from build123d import *

# Parameters (mm, degrees)
BOSS_EXTRUDE1_DEPTH   = 30
FILLET1_R             = 10
CHAMFER1_SIZE         = 2
SKETCH3_R             = 1.9
CUT_EXTRUDE1_DEPTH    = 32.825
CHAMFER2_SIZE         = 2
CHAMFER2_SIZE2        = 0.352653961
CHAMFER2_PART_2_SIZE  = 2
CHAMFER2_PART_2_SIZE2 = 0.352653961
CHAMFER2_PART_3_SIZE  = 2
CHAMFER2_PART_3_SIZE2 = 0.352653961
CHAMFER2_PART_4_SIZE  = 2
CHAMFER2_PART_4_SIZE2 = 0.352653961


with BuildPart() as part:
    # Sketch1 → Boss-Extrude1 (new body)
    with BuildSketch(Plane.XY):
        with BuildLine():
            Line((0, 3.175), (0, 0))
            ThreePointArc((0, 0), (10.672667654, 4.397249215), (15.150137433, 15.036511402))
            ThreePointArc((15.150137433, 15.036511402), (20.018255831, 19.849965642), (24.85, 15))
            Line((24.85, 15), (24.85, 7.575))
            ThreePointArc((24.85, 7.575), (32.425, 0), (40, 7.575))
            Line((40, 7.575), (40, 15))
            ThreePointArc((40, 15), (25.241541186, 34.300938992), (2.747375401, 25.116666667))
            ThreePointArc((2.747375401, 25.116666667), (-0.908189135, 21.497922919), (-5.878936899, 20.175))
            Line((-5.878936899, 20.175), (-40, 20.175))
            Line((-40, 20.175), (-40, 3.175))
            Line((-40, 3.175), (0, 3.175))
        make_face()
    extrude(amount=BOSS_EXTRUDE1_DEPTH)

    # Fillet1
    fillet1_edges = [part.edges().sort_by_distance(p)[0] for p in [
        (-40, 11.675, 0),
        (-40, 11.675, 30),
    ]]
    fillet(fillet1_edges, radius=FILLET1_R)

    # Chamfer1
    chamfer1_edges = [part.edges().sort_by_distance(p)[0] for p in [
        (-17.939468449, 20.175, 0),
        (-0.908189135, 21.497922919, 0),
        (25.241541186, 34.300938992, 0),
        (40, 11.2875, 0),
        (10.672667654, 4.397249215, 30),
        (32.425, 0, 0),
        (24.85, 11.2875, 0),
        (20.018255831, 19.849965642, 0),
        (10.672667654, 4.397249215, 0),
        (0, 1.5875, 0),
        (20.018255831, 19.849965642, 30),
        (24.85, 11.2875, 30),
        (32.425, 0, 30),
        (40, 11.2875, 30),
        (25.241541186, 34.300938992, 30),
        (-40, 3.175, 15),
        (-40, 20.175, 15),
        (-15, 3.175, 0),
        (-15, 3.175, 30),
        (-37.071067812, 3.175, 27.071067812),
        (-0.908189135, 21.497922919, 30),
        (-37.071067812, 3.175, 2.928932188),
        (-37.071067812, 20.175, 27.071067812),
        (-37.071067812, 20.175, 2.928932188),
        (-17.939468449, 20.175, 30),
        (0, 1.5875, 30),
    ]]
    chamfer(chamfer1_edges, length=CHAMFER1_SIZE)

    # Sketch3 → Cut-Extrude1 (cut, through all)
    with BuildSketch(Plane.XZ.offset(-3.175)):
        with Locations((-30, 20)):
            Circle(SKETCH3_R)
        with Locations((-15, 20)):
            Circle(SKETCH3_R)
        with Locations((-15, 10)):
            Circle(SKETCH3_R)
        with Locations((-30, 10)):
            Circle(SKETCH3_R)
    extrude(amount=-CUT_EXTRUDE1_DEPTH, mode=Mode.SUBTRACT)

    # Chamfer2
    chamfer2_edges = [part.edges().sort_by_distance(p)[0] for p in [
        (-31.9, 3.175, 10),
    ]]
    chamfer2_side = [part.faces().sort_by_distance(p)[0] for p in [
        (-31.9, 11.675, 10),
    ]]
    chamfer(chamfer2_edges, length=CHAMFER2_SIZE, length2=CHAMFER2_SIZE2, reference=chamfer2_side[0])

    # Chamfer2 part 2
    chamfer2_part_2_edges = [part.edges().sort_by_distance(p)[0] for p in [
        (-16.9, 3.175, 10),
    ]]
    chamfer2_part_2_side = [part.faces().sort_by_distance(p)[0] for p in [
        (-16.9, 11.675, 10),
    ]]
    chamfer(chamfer2_part_2_edges, length=CHAMFER2_PART_2_SIZE, length2=CHAMFER2_PART_2_SIZE2, reference=chamfer2_part_2_side[0])

    # Chamfer2 part 3
    chamfer2_part_3_edges = [part.edges().sort_by_distance(p)[0] for p in [
        (-16.9, 3.175, 20),
    ]]
    chamfer2_part_3_side = [part.faces().sort_by_distance(p)[0] for p in [
        (-16.9, 11.675, 20),
    ]]
    chamfer(chamfer2_part_3_edges, length=CHAMFER2_PART_3_SIZE, length2=CHAMFER2_PART_3_SIZE2, reference=chamfer2_part_3_side[0])

    # Chamfer2 part 4
    chamfer2_part_4_edges = [part.edges().sort_by_distance(p)[0] for p in [
        (-31.9, 3.175, 20),
    ]]
    chamfer2_part_4_side = [part.faces().sort_by_distance(p)[0] for p in [
        (-31.9, 11.675, 20),
    ]]
    chamfer(chamfer2_part_4_edges, length=CHAMFER2_PART_4_SIZE, length2=CHAMFER2_PART_4_SIZE2, reference=chamfer2_part_4_side[0])


solid = part.part
Read the model definition and answer for the solid it produces. Units are mm, in the model's axes. A direction names the side the tool comes from. Coordinates: 2 decimals unless noted, no trailing zeros. Write each loop counter-clockwise with the first axis right and the second up, starting at its lowest first coordinate (ties: lowest second). Pieces come first, ordered by that corner, then holes. Notation, with made-up numbers: (23.25, 24.25) -> (70.25, 24.25) arc R14 ccw to (70.25, 46.25) -> close; hole circle Ø10 at (71.25, -24). An arc over 180 degrees is marked (long way). Return JSON: item names as keys, results as strings.
(1) Consider line 1 along Z through (x, y) = (-15, 10.25); line 2 along Y through (x, z) = (-35, 7.5) (3 decimals); line 3 along X through (y, z) = (18, 26.5). Determine where each line is inside the solid, lowest interval first. Write a range as from..to.
Answers below:
{"line 1": "0..8.1, 11.9..18.1, 21.9..30", "line 2": "3.175..20.175", "line 3": "-37.6..16.19, 23.81..39.77"}
(2) The part is cut by section C-C on x = 20. Give the vertices of the cut face in (y, z).
Answers below:
{"outline": "(19.85, 2) -> (21.85, 0) -> (33, 0) -> (35, 2) -> (35, 28) -> (33, 30) -> (21.85, 30) -> (19.85, 28) -> close"}
(3) The part is cut by section D-D on y = 13. State how many separate pieces and enclosed holes the cut face has, then the cut area to 3 significant figures.
Answers below:
{"separate pieces": "2", "enclosed holes": "4", "area": "2,000 mm^2"}
(4) For a pull along Z with two mould halves and no side action, classify faces 1 (the flat face through (40, 11, 15)), 2 (the conical face through (-28.092, 4.605, 10.601)), 3 (the conical face through (-35.97, 3.72, 3.89)) as pulls with the +Z half, pulls with the -Z half, needs draft (parallel to the pull), parting line crosses it, or undercut.
Answers below:
{"face 1": "needs draft", "face 2": "undercut", "face 3": "pulls with the -Z half"}
(5) Which of the six approach directions +Z, -Z, +X, -X, +Y, -Y give full straight-line access (tool end or side, diameter ignored) to faces 4 (the flat face through (25.86, 11.24, 29.01)), 5 (the cylindrical face through (10.554, 4.281, 14.818)), 6 (the flat face through (0, 2, 15)), 7 (the flat face through (1, 3, 29)), 8 (the flat face through (-22, 20.175, 15))?
Answers below:
{"face 4": "+Z, -Y", "face 5": "+Z, -Z, -Y", "face 6": "+Z, -Z, -X, -Y", "face 7": "+Z, -X, -Y", "face 8": "+Z, -Z, -X, +Y"}
(6) The part is cut by section B-B on z = 13. Give the vertices of the cut face in (x, y) (3 decimals).
Answers below:
{"outline": "(-40, 5.175) -> (-38, 3.175) -> (0, 3.175) -> (0, 0) arc R15.151 ccw to (15.15, 15.037) arc R4.85 cw to (24.85, 15) -> (24.85, 7.575) arc R7.575 ccw to (40, 7.575) -> (40, 15) arc R20 ccw to (2.747, 25.117) arc R10 cw to (-5.879, 20.175) -> (-38, 20.175) -> (-40, 18.175) -> close"}
(7) The part is cut by section A-A on x = -15. Give the vertices of the cut face in (y, z) (3 decimals), then the cut area to 3 significant figures.
Answers below:
{"outline": "(3.175, 2) -> (5.175, 0) -> (18.175, 0) -> (20.175, 2) -> (20.175, 8.1) -> (5.175, 8.1) -> (3.175, 7.747) -> close; (3.175, 12.253) -> (5.175, 11.9) -> (20.175, 11.9) -> (20.175, 18.1) -> (5.175, 18.1) -> (3.175, 17.747) -> close; (3.175, 22.253) -> (5.175, 21.9) -> (20.175, 21.9) -> (20.175, 28) -> (18.175, 30) -> (5.175, 30) -> (3.175, 28) -> close", "area": "371 mm^2"}
(8) Each of these flat-tipped pins is pushed along its axis until it touches: P1, Ø2, axis at x = -16.5, z = 23, coming from the +Y side (3 decimals); P2, Ø3, axis at y = 20, z = 25.5, coming from the -X side; P3, Ø1, axis at y = 8.5, z = 6.5, coming from the -X side; P4, Ø3, axis at x = -15, z = 20, coming from the -Y side. Where does it stop, or does it pass through?
Answers below:
{"P1": "y = 20.175", "P2": "x = -38.2", "P3": "x = -39.54", "P4": "through"}
